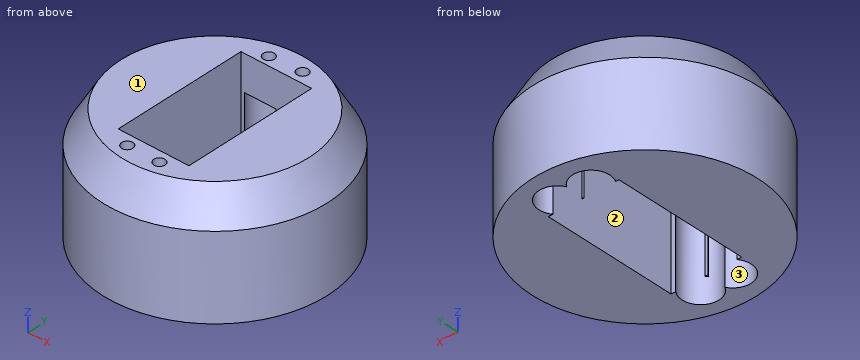
```python
from build123d import *

# Parameters (mm, degrees)
SKETCH1_R           = 35
BOSS_EXTRUDE1_DEPTH = 36
CHAMFER1_SIZE       = 10
CHAMFER1_SIZE2      = 5.773502692
SKETCH2_W           = 22
SKETCH2_H           = 42
CUT_EXTRUDE1_DEPTH  = 37
SKETCH3_R           = 1.75
CUT_EXTRUDE2_DEPTH  = 37
SKETCH4_R           = 1.75
CUT_EXTRUDE3_DEPTH  = 25


with BuildPart() as part:
    # Sketch1 → Boss-Extrude1 (new body)
    with BuildSketch(Plane.XY):
        Circle(SKETCH1_R)
    extrude(amount=BOSS_EXTRUDE1_DEPTH)

    # Chamfer1
    chamfer1_edges = [part.edges().sort_by_distance(p)[0] for p in [
        (-35, 0, 36),
    ]]
    chamfer1_side = [part.faces().sort_by_distance(p)[0] for p in [
        (-35, 0, 18),
    ]]
    chamfer(chamfer1_edges, length=CHAMFER1_SIZE, length2=CHAMFER1_SIZE2, reference=chamfer1_side[0])

    # Sketch2 → Cut-Extrude1 (cut, through all)
    with BuildSketch(Plane.XY.offset(36)):
        Rectangle(SKETCH2_W, SKETCH2_H)
    extrude(amount=-CUT_EXTRUDE1_DEPTH, mode=Mode.SUBTRACT)

    # Sketch3 → Cut-Extrude2 (cut, through all)
    with BuildSketch(Plane.XY.offset(36)):
        with Locations((-5, 23.927118757)):
            Circle(SKETCH3_R)
        with Locations((5, 24.5)):
            Circle(SKETCH3_R)
        with Locations((5, -24.5)):
            Circle(SKETCH3_R)
        with Locations((-5, -24.5)):
            Circle(SKETCH3_R)
    extrude(amount=-CUT_EXTRUDE2_DEPTH, mode=Mode.SUBTRACT)

    # Sketch4 → Cut-Extrude3 (cut)
    with BuildSketch(Plane(origin=(0, 0, 0), x_dir=(-1, 0, 0), z_dir=(0, 0, -1))):
        with BuildLine():
            ThreePointArc((0, -21.660545827), (-10.75, -24.5), (0, -27.339454173))
            ThreePointArc((0, -27.339454173), (10.75, -24.5), (0, -21.660545827))
        make_face()
        with Locations((-5, -24.5)):
            Circle(SKETCH4_R, mode=Mode.SUBTRACT)
        with Locations((5, -24.5)):
            Circle(SKETCH4_R, mode=Mode.SUBTRACT)
        with BuildLine():
            ThreePointArc((-0.161572278, 21.393214334), (10.740587615, 23.59825126), (0.161572278, 27.033904423))
            ThreePointArc((0.161572278, 27.033904423), (-10.740587615, 24.828867497), (-0.161572278, 21.393214334))
        make_face()
        with Locations((5, 23.927118757)):
            Circle(SKETCH4_R, mode=Mode.SUBTRACT)
        with Locations((-5, 24.5)):
            Circle(SKETCH4_R, mode=Mode.SUBTRACT)
    extrude(amount=-CUT_EXTRUDE3_DEPTH, mode=Mode.SUBTRACT)


solid = part.part
```
Source: CAD feature listing. Evaluate the final solid. Frame: model axes, mm. Face numbers are marked on the shaded views. A direction names the side the tool comes from. Give positions to 0.01 mm unless a question says otherwise; leave off trailing zeros. Loops run counter-clockwise (first coordinate to the right, second up) from the corner with the lowest first, then second, coordinate; pieces in that order, holes last. Notation, with made-up numbers: (39, -27.5) - (85, -27.5) arc R7 ccw to (85, -16.5) - close; hole circle Ø10 at (-6, 23.25). An arc over 180 degrees is marked (long way). Use CSV: the item, a comma, the result in double quotes. Start each with the question number.
1. Ray query, L1, parallel to X at y = -24.5, z = 30; L2, parallel to Y at x = -5, z = 27.5; L3, parallel to X at y = -23, z = 34. Return the intervals inside material, ascending.
2. Section C-C (z = 29). Output: boundary loops of the cut face in (x, y).
3. Pin query (flat end, axial travel): pin 1 (3 mm diameter, centred on x = 9.5, z = 13.5, fed in from -Y); pin 2 (4 mm diameter, centred on x = 5, y = -24.5, fed in from -Z); pin 3 (2 mm diameter, centred on y = 5.5, z = 28, fed in from -X). Return the tip coordinate at first contact, or that it passes through.
4. Section A-A (y = 0). Output: boundary loops of the cut face in (x, z).
5. Section B-B (z = 10.5). Output: boundary loops of the cut face in (x, y).
6. Reachability of the marked faces 1, 2 and 3 from +Z, -Z, +X, -X, +Y, -Y: full face, straight path, thin tool, end or side. Return the list, or none.
7. Section D-D (y = -24.5). Count the separate pieces of the cut face and the enclosed holes in it, then the cut area to 3 significant figures.
Response:
1,L1,"-21.64 to -6.75, -3.25 to 3.25, 6.75 to 21.64"
1,L2,"-33.77 to -26.25, -22.75 to -21, 21 to 22.18, 25.68 to 33.77"
1,L3,"-19.85 to -5.9, -4.1 to 4.1, 5.9 to 19.85"
2,outline,"circle Ø66.54 at (0, 0); hole (-11, -21) - (11, -21) - (11, 21) - (-11, 21) - close; hole circle Ø3.5 at (-5, -24.5); hole circle Ø3.5 at (-5, 23.93); hole circle Ø3.5 at (5, -24.5); hole circle Ø3.5 at (5, 24.5)"
3,pin 1,"y = -34.07"
3,pin 2,"z = 25"
3,pin 3,"x = -34"
4,outline,"(-35, 0) - (-11, 0) - (-11, 36) - (-29.23, 36) - (-35, 26) - close; (11, 0) - (35, 0) - (35, 26) - (29.23, 36) - (11, 36) - close"
5,outline,"circle Ø70 at (0, 0); (-0.44, -21) arc R5.75 cw to (0, -21.66) arc R5.75 cw to (0.44, -21) - close; (-0.05, 21) - (0.44, 21) arc R5.75 cw to (0.16, 21.39) arc R5.75 cw to start; hole (-11, -21) - (-9.56, -21) arc R5.75 ccw (long way) to (0, -27.34) arc R5.75 ccw (long way) to (9.56, -21) - (11, -21) - (11, 21) - (9.56, 21) arc R5.75 ccw (long way) to (-0.16, 27.03) arc R5.75 ccw to (-9.95, 21) - (-11, 21) - close"
6,face 1,"+Z, +X, -X, +Y, -Y"
6,face 2,"+Z, -Z"
6,face 3,"-Z"
7,separate pieces,"3"
7,enclosed holes,"0"
7,area,"1,100 mm²"
